Design review of the part built by this model. Coordinates are the model's own, in mm. Face numbers are marked on the shaded views. A direction names the side the tool comes from. Give positions to 0.01 mm unless a question says otherwise; leave off trailing zeros. Loops run counter-clockwise (first coordinate to the right, second up) from the corner with the lowest first, then second, coordinate; pieces in that order, holes last. Notation, with made-up numbers: (-27.75, 40) -> (-0.75, 40) arc R28 ccw to (-0.75, 79) -> close; hole circle Ø10 at (-36, 64). An arc over 180 degrees is marked (long way). Use CSV: the item, a comma, the result in double quotes. Start each with the question number.
Item 1: Wall thickness on line 1 along X through (y, z) = (402, 1); line 2 along Y through (x, z) = (-4, -18): over which ranges is each line inside the solid? List them lowest first. Write a range as from..to.
Item 2: We need section A-A (z = 0). State the section outline as (x, y) points, plus the area to 3 significant figures.
Item 3: For the marked faces 1 and 2, list the 3-axis set-ups (+Z, -Z, +X, -X, +Y, -Y) from which the entire face can be reached by the end or side of a thin tool; tool diameter is ignored.
Item 4: Clearance check with flat-ended pins moving along their axes: pin 1 (1.5 mm diameter, centred on x = 4.5, z = -11.5, fed in from +Y); pin 2 (22 mm diameter, centred on x = 0, y = 206, fed in from +Z); pin 3 (12 mm diameter, centred on y = 413, z = -10.5, fed in from -X); pin 4 (3 mm diameter, centred on x = -12.5, y = 182, fed in from -Z). State where each tip first meets the part, or that it passes through.
Item 5: We need section B-B (y = 441). State the section outline as (x, z) points.
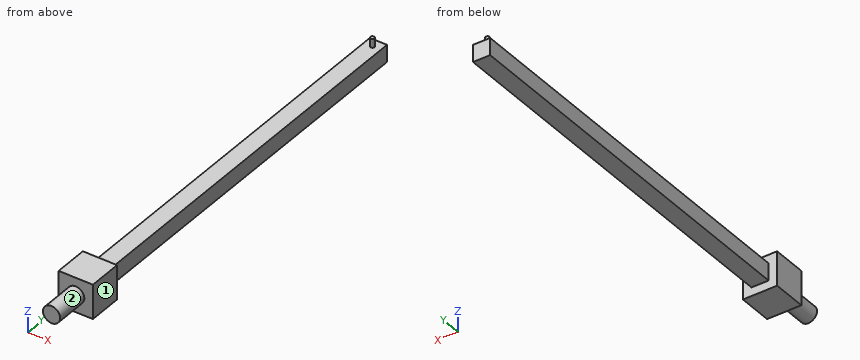
from build123d import *

# Parameters (mm, degrees)
SKETCH1_W           = 20
SKETCH1_H           = 20
BOSS_EXTRUDE1_DEPTH = 500
SKETCH2_W           = 40
SKETCH2_H           = 40
BOSS_EXTRUDE2_DEPTH = 40
SKETCH3_R           = 10
BOSS_EXTRUDE3_DEPTH = 40
SKETCH4_R           = 2.5
BOSS_EXTRUDE4_DEPTH = 10


with BuildPart() as part:
    # Sketch1 → Boss-Extrude1 (new body)
    with BuildSketch(Plane(origin=(0, 0, 0), x_dir=(1, 0, 0), z_dir=(0, 1, 0))):
        Rectangle(SKETCH1_W, SKETCH1_H)
    extrude(amount=BOSS_EXTRUDE1_DEPTH)

    # Sketch2 → Boss-Extrude2 (add)
    with BuildSketch(Plane.XZ):
        Rectangle(SKETCH2_W, SKETCH2_H)
    extrude(amount=-BOSS_EXTRUDE2_DEPTH)

    # Sketch3 → Boss-Extrude3 (add)
    with BuildSketch(Plane.XZ):
        Circle(SKETCH3_R)
    extrude(amount=BOSS_EXTRUDE3_DEPTH)

    # Sketch4 → Boss-Extrude4 (add)
    with BuildSketch(Plane.XY.offset(10)):
        with Locations((0, 490)):
            Circle(SKETCH4_R)
    extrude(amount=BOSS_EXTRUDE4_DEPTH)


solid = part.part
Results found:
1,line 1,"-10..10"
1,line 2,"0..40"
2,outline,"(-20, 0) -> (-10, 0) -> (-10, -40) -> (10, -40) -> (10, 0) -> (20, 0) -> (20, 40) -> (10, 40) -> (10, 500) -> (-10, 500) -> (-10, 40) -> (-20, 40) -> close"
2,area,"11,600 mm²"
3,face 1,"+Z, -Z, +X, +Y, -Y"
3,face 2,"-Y"
4,pin 1,"y = 40"
4,pin 2,"z = 10"
4,pin 3,"x = -10"
4,pin 4,"through"
5,outline,"(-10, -10) -> (10, -10) -> (10, 10) -> (-10, 10) -> close"
